Geometry: final body of the model. Coordinates: model frame, mm. Face numbers are marked on the shaded views. A direction names the side the tool comes from. Coordinates: 2 decimals unless noted, no trailing zeros. Order: outer loops, then holes, each group sorted by start corner. A loop starts at its lowest first (then second) coordinate and runs counter-clockwise, first axis right, second up. Notation, with made-up numbers: M 72,-23.75 L 84,-23.75 A21 ccw 84,-15.75 Z; hole C 61.5,8 d3. An arc over 180 degrees is marked long. Use CSV: the item, a comma, the result in double quotes. Start each with the question number.
Q1. Section query D-D, the plane x = 12. Output: boundary loops of the cut face in (y, z), and give its area (3 significant figures).
Q2. Section query C-C, the plane z = 0.75. Output: boundary loops of the cut face in (x, y).
Q3. Section query B-B, the plane y = -3.5. Output: boundary loops of the cut face in (x, z).
Q4. Ray query, probe 1 along Z at (x, y) = (-20, -22); probe 2 along Y at (x, z) = (3, -8); probe 3 along X at (y, z) = (-29, -9). Return the intervals inside material, ascending.
Q5. Access query for the marked faces 1, 2 and 3. Directions: +Z, -Z, +X, -X, +Y, -Y. A direction counts if a zero-diameter tool reaches every point of the face in a straight line with its end or side. Return the directions, or none.
Q6. Section query A-A, the plane x = 7.5. Output: boundary loops of the cut face in (y, z).
Q7. First-contact query: P1, Ø3, axis at x = -15.5, y = -9, coming from the -Z side; P2, Ø0.6, axis at x = -4, z = 1, coming from the +Y side; P3, Ø4, axis at x = -11, z = -4.5, coming from the +Y side; P4, Ø8, axis at x = -3.5, z = -5, coming from the -Y side. Flat tips, straight axial feed; report the tip coordinate or a pass-through.
Autodesk Inventor part; units mm, degrees
ref_plane "YZ Plane" through (0, 0, 0) normal (1, 0, 0) x (0, 1, 0)
ref_plane "XZ Plane" through (0, 0, 0) normal (0, 1, 0) x (-1, 0, 0)
ref_plane "XY Plane" through (0, 0, 0) normal (0, 0, 1) x (1, 0, 0)
sketch "Sketch1" plane through (0, 0, 0) normal (0, 0, 1) x (1, 0, 0)
  line L0 (-28.7318, -0.5685) -> (-18.7318, -0.5685)
  line L1 (-18.7318, -0.5685) -> (-18.7318, -30.5685)
  line L2 (-18.7318, -30.5685) -> (-28.7318, -30.5685)
  line L3 (-28.7318, -30.5685) -> (-28.7318, -0.5685)
  line L4 (-28.7318, -30.5685) -> (16.2682, -30.5685)
  line L5 (16.2682, -30.5685) -> (16.2682, -20.5685)
  line L6 (16.2682, -20.5685) -> (-28.7318, -20.5685)
  line L7 (-28.7318, -20.5685) -> (-28.7318, -30.5685)
  line L8 (16.2682, -30.5685) -> (6.2682, -30.5685)
  line L9 (6.2682, -30.5685) -> (6.2682, -0.5685)
  line L10 (6.2682, -0.5685) -> (16.2682, -0.5685)
  line L11 (16.2682, -0.5685) -> (16.2682, -30.5685)
  circle A0 centre (-23.7318, -4.6959) radius 2
  circle A1 centre (11.2682, -4.6959) radius 2
  point P0 (0, 0)
  dimension "d0" = 45
  dimension "d1" = 10
  dimension "d2" = 10
  dimension "d3" = 10
  dimension "d4" = 30
  dimension "d5" = 4
  dimension "d6" = 4
extrude "Extrusion1" add sketch "Sketch1" along normal blind 2
fillet "Fillet1" radius 5 2 edges at (-18.7318, -20.5685, 1) (6.2682, -20.5685, 1)
sketch "Sketch2" plane through (0, 0, 0) normal (0, 0, -1) x (-1, 0, 0)
  line L0 (28.7318, -0.5685) -> (28.7318, -30.5685)
  line L1 (-16.1665, -30.4376) -> (28.7318, -30.4376)
  line L2 (28.7318, -30.4376) -> (28.7318, -28.4376)
  line L3 (28.7318, -28.4376) -> (-16.1665, -28.4376)
  line L4 (-16.1665, -28.4376) -> (-16.1665, -30.4376)
  point P0 (0, 0)
  dimension "d10" = 2
extrude "Extrusion2" add sketch "Sketch2" along normal blind 20
fillet "Fillet2" radius 2 1 edges at (-6.2826, -28.4376, 0)
properties part number "stpper holder"
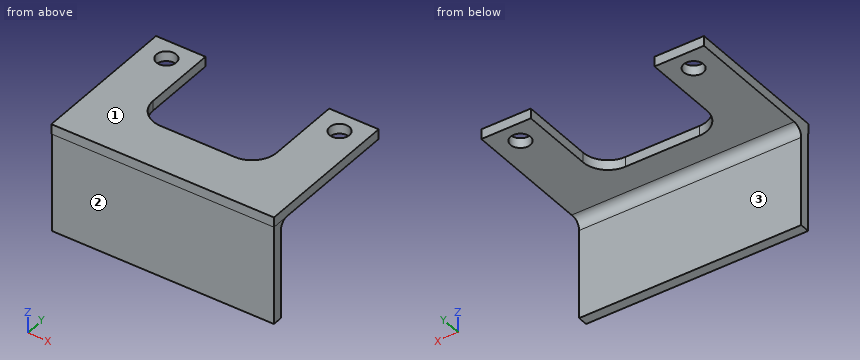
Responses:
1,outline,"M -30.57,0 L -30.44,0 L -30.44,-20 L -28.44,-20 L -28.44,-2 A2 cw -26.44,0 L -6.56,0 L -6.56,2 L -30.57,2 Z; M -2.83,0 L -0.57,0 L -0.57,2 L -2.83,2 Z"
1,area,"93.4 mm²"
2,outline,"M -28.73,-30.57 L 16.27,-30.57 L 16.27,-0.57 L 6.27,-0.57 L 6.27,-15.57 A5 cw 1.27,-20.57 L -13.73,-20.57 A5 cw -18.73,-15.57 L -18.73,-0.57 L -28.73,-0.57 Z; hole C -23.73,-4.7 d4; hole C 11.27,-4.7 d4"
3,outline,"M -28.73,0 L -25.33,0 L -25.33,2 L -28.73,2 Z; M -22.13,0 L -18.73,0 L -18.73,2 L -22.13,2 Z; M 6.27,0 L 9.67,0 L 9.67,2 L 6.27,2 Z; M 12.87,0 L 16.27,0 L 16.27,2 L 12.87,2 Z"
4,probe 1,"z = 0 to 2"
4,probe 2,"y = -30.44 to -28.44"
4,probe 3,"x = -28.73 to 16.17"
5,face 1,"+Z, +X, -X, +Y, -Y"
5,face 2,"-Z, +X, -X, -Y"
5,face 3,"-Z, +X, -X, +Y"
6,outline,"M -30.57,0 L -30.44,0 L -30.44,-20 L -28.44,-20 L -28.44,-2 A2 cw -26.44,0 L -0.57,0 L -0.57,2 L -30.57,2 Z"
7,P1,"passes through"
7,P2,"stops at y = -20.57"
7,P3,"stops at y = -28.44"
7,P4,"stops at y = -30.44"
